```python
from build123d import *

# Parameters (mm, degrees)
F0_R     = 2.25
F0_R_2   = 2
F1_DEPTH = 2.5
F2_R     = 2


with BuildPart() as f1:
    # F0 (on Front) → F1 (new body, symmetric)
    with BuildSketch(Plane.XZ):
        with BuildLine():
            ThreePointArc((3.5986671115, -2.7017762714), (4.2687235798, -1.4240782981), (4.5, 0))
            ThreePointArc((4.5, 0), (4.2687235798, 1.4240782981), (3.5986671115, 2.7017762714))
            ThreePointArc((3.5986671115, 2.7017762714), (-4.5, 0), (3.5986671115, -2.7017762714))
        make_face()
        Circle(F0_R, mode=Mode.SUBTRACT)
        with BuildLine():
            ThreePointArc((3.5986671115, 2.7017762714), (4.2687235798, 1.4240782981), (4.5, 0))
            ThreePointArc((4.5, 0), (4.2687235798, -1.4240782981), (3.5986671115, -2.7017762714))
            Line((3.5986671115, -2.7017762714), (96.4013328885, -2.7017762714))
            ThreePointArc((96.4013328885, -2.7017762714), (95.5, 0), (96.4013328885, 2.7017762714))
            Line((96.4013328885, 2.7017762714), (3.5986671115, 2.7017762714))
        make_face()
        with BuildLine():
            ThreePointArc((104.5, 0), (101.4240782981, 4.2687235798), (96.4013328885, 2.7017762714))
            ThreePointArc((96.4013328885, 2.7017762714), (95.5, 0), (96.4013328885, -2.7017762714))
            ThreePointArc((96.4013328885, -2.7017762714), (101.4240782981, -4.2687235798), (104.5, 0))
        make_face()
        with Locations((100, 0)):
            Circle(F0_R_2, mode=Mode.SUBTRACT)
    extrude(amount=F1_DEPTH, both=True)

    # F2
    f2_edges = [f1.edges().sort_by_distance(p)[0] for p in [
        (3.598667, 0, 2.701776),
        (96.401333, 0, 2.701776),
        (3.598667, 0, -2.701776),
        (96.401333, 0, -2.701776),
    ]]
    fillet(f2_edges, radius=F2_R)


solid = f1.part
```
Check sheet for the modelled part. Datum: model origin and axes. Units: mm. A direction names the side the tool comes from. Coordinates: 2 decimals unless noted, no trailing zeros. Write each loop counter-clockwise with the first axis right and the second up, starting at its lowest first coordinate (ties: lowest second). Pieces come first, ordered by that corner, then holes. Notation, with made-up numbers: (62, 46.25) - (100, 46.25) arc R24 cw to (100, 75.25) - close; hole circle Ø2 at (-13, 77.25). An arc over 180 degrees is marked (long way). One line per question, with ' | ' between items.
Item 1: Thickness scan on line 1 (Z direction, x = 0, y = 0.35); line 2 (Z direction, x = 100, y = -0.95); line 3 (X direction, y = 1.65, z = 0.5). Record the ranges inside material, lowest first. Write a range as [from, to].
Determined:
line 1: z = [-4.5, -2.25], [2.25, 4.5] | line 2: z = [-4.5, -2], [2, 4.5] | line 3: x = [-4.47, -2.19], [2.19, 98.06], [101.94, 104.47]
Item 2: Sectioned sample at D-D on x = 100. Record the boundary of the cut face in (y, z).
Determined:
outline: (-2.5, -4.5) - (2.5, -4.5) - (2.5, -2) - (-2.5, -2) - close; (-2.5, 2) - (2.5, 2) - (2.5, 4.5) - (-2.5, 4.5) - close
Item 3: Sectioned sample at B-B on y = -0.3. Record the boundary of the cut face in (x, z).
Determined:
outline: (3.11, -3.26) arc R2 cw to (4.49, -2.7) - (95.51, -2.7) arc R2 cw to (96.89, -3.26) arc R4.5 ccw (long way) to (96.89, 3.26) arc R2 cw to (95.51, 2.7) - (4.49, 2.7) arc R2 cw to (3.11, 3.26) arc R4.5 ccw (long way) to start; hole circle Ø4.5 at (0, 0); hole circle Ø4 at (100, 0)
Item 4: Sectioned sample at A-A on z = 0. Record the boundary of the cut face in (x, y).
Determined:
outline: (-4.5, -2.5) - (-2.25, -2.5) - (-2.25, 2.5) - (-4.5, 2.5) - close; (2.25, -2.5) - (98, -2.5) - (98, 2.5) - (2.25, 2.5) - close; (102, -2.5) - (104.5, -2.5) - (104.5, 2.5) - (102, 2.5) - close
Item 5: Mould release check, pull along Z, two halves, no side actions. Record for faces 3 (the face through (51, 0, 2.702)), 4 (the face through (101.908, 0.035, 0.601)), 5 (the face through (104.5, 0, -0.1)): pulls with the +Z half, pulls with the -Z half, needs draft (parallel to the pull), parting line crosses it, or undercut.
Determined:
face 3: pulls with the +Z half | face 4: undercut | face 5: parting line crosses it
Item 6: Gauge pin test, flat ends, axial feed: P1, Ø3, axis at x = 81.5, y = 0.5, coming from the +Z side; P2, Ø2, axis at x = 41, y = 1, coming from the -Z side; P3, Ø2, axis at y = 1, z = -2, coming from the -X side. Record the tip position at first contact, or that the pin passes through.
Determined:
P1: stops at z = 2.7 | P2: stops at z = -2.7 | P3: stops at x = -4.39
Item 7: Access from +Z, -Z, +X, -X, +Y, -Y to the whole of each face (thin tool, end or side, straight path). Record for faces 1 (the face through (49, -2.5, 0)), 2 (the face through (49, 0, -2.702)).
Determined:
face 1: +Z, -Z, +X, -X, -Y | face 2: -Z, +Y, -Y
Item 8: Sectioned sample at C-C on x = 0. Record the boundary of the cut face in (y, z).
Determined:
outline: (-2.5, -4.5) - (2.5, -4.5) - (2.5, -2.25) - (-2.5, -2.25) - close; (-2.5, 2.25) - (2.5, 2.25) - (2.5, 4.5) - (-2.5, 4.5) - close
